Autodesk Inventor part; units mm, degrees
ref_plane "YZ Plane" through (0, 0, 0) normal (1, 0, 0) x (0, 1, 0)
ref_plane "XZ Plane" through (0, 0, 0) normal (0, 1, 0) x (-1, 0, 0)
ref_plane "XY Plane" through (0, 0, 0) normal (0, 0, 1) x (1, 0, 0)
sketch "Sketch1" plane through (0, 0, 0) normal (0, 1, 0) x (-1, 0, 0)
  line L0 (10.6592, 63.5) -> (-7.8828, 63.5)
  line L1 (-7.8828, 63.5) -> (-7.8828, -12.7)
  line L2 (-7.8828, -12.7) -> (10.6592, -12.7)
  line L3 (10.6592, 57.785) -> (-1.5328, 57.785)
  line L4 (-1.5328, 57.785) -> (-1.5328, 31.75)
  line L5 (-1.5328, 31.75) -> (10.6592, 31.75)
  line L6 (10.6592, 19.05) -> (-1.5328, 19.05)
  line L7 (-1.5328, 19.05) -> (-1.5328, -6.35)
  line L8 (-1.5328, -6.35) -> (10.6592, -6.35)
  line L9 (10.6592, -12.7) -> (10.6592, -6.35)
  line L10 (10.6592, 19.05) -> (10.6592, 31.75)
  line L11 (10.6592, 57.785) -> (10.6592, 63.5)
  point P0 (0, 0)
  dimension "d0" = 18.542
  dimension "d3" = 6.35
  dimension "d4" = 12.7
  dimension "d5" = 5.715
  dimension "d7" = 0
  dimension "d8" = 26.035
  dimension "d9" = 25.4
  dimension "d25" = 0
  dimension "d26" = 0
extrude "Extrusion1" add sketch "Sketch1" along normal blind 101.6
sketch "Sketch2" plane through (1.5328, 0, -6.35) normal (-1, 0, 0) x (0, 0, 1)
  line L0 (0, 0) -> (0, 101.6)
  line L1 (0, 0) -> (25.4, 0)
  point P0 (6.35, 0)
  point P1 (12.7, 25.4)
  point P2 (12.7, 50.8)
  point P3 (12.7, 76.2)
  dimension "d12" = 12.7
  dimension "d13" = 25.4
  dimension "d14" = 25.4
  dimension "d15" = 0
  dimension "d16" = 0
  dimension "d17" = 25.4
hole "Hole1" at (1.5328, 25.4, 6.35) at (1.5328, 50.8, 6.35) at (1.5328, 76.2, 6.35) direction (1, 0, 0) diameter 4.826 depth 25.4 tip angle 118
sketch "Sketch3" plane through (0, 101.6, 0) normal (0, 1, 0) x (1, 0, 0)
  line L0 (1.5328, -31.75) -> (-10.7917, -31.3196)
  line L1 (-10.7917, -31.3196) -> (-10.7917, -31.75)
  line L2 (-10.6592, -31.75) -> (1.5328, -31.75)
  line L3 (-10.7917, -31.75) -> (1.5328, -31.75)
  point P0 (0, 0)
  dimension "d27" = 2
extrude "Extrusion2" cut sketch "Sketch3" against normal blind 111.125
sketch "Sketch4" plane through (0, 101.6, 0) normal (0, 1, 0) x (1, 0, 0)
  line L0 (1.5328, -57.785) -> (-12.9577, -57.785)
  line L1 (-12.9577, -57.785) -> (-12.9577, -58.291)
  line L2 (-12.9577, -58.291) -> (1.5328, -57.785)
  point P0 (0, 0)
  dimension "d30" = 2
extrude "Extrusion3" cut sketch "Sketch4" against normal blind 119.0625
sketch "Sketch5" plane through (0, 101.6, 0) normal (0, 1, 0) x (1, 0, 0)
  line L0 (-10.6592, -63.5) -> (7.8828, -63.5)
  line L1 (7.8828, -63.5) -> (-13.0423, -62.7693)
  line L2 (-13.0423, -62.7693) -> (-13.0009, -63.5)
  line L3 (-13.0009, -63.5) -> (7.8828, -63.5)
  point P0 (0, 0)
  dimension "d33" = 2
extrude "Extrusion4" cut sketch "Sketch5" against normal blind 196.85
sketch "Sketch6" plane through (0, 101.6, 0) normal (0, 1, 0) x (1, 0, 0)
  line L0 (7.8828, 12.7) -> (-10.6592, 12.7)
  line L1 (7.8828, 12.7) -> (-16.8119, 12.7)
  line L2 (-16.8119, 12.7) -> (-16.8119, 11.8376)
  line L3 (7.8828, -63.5) -> (7.8828, 12.7)
  line L4 (-16.8119, 11.8376) -> (7.8828, 12.7)
  point P0 (0, 0)
  dimension "d36" = 2
extrude "Extrusion5" cut sketch "Sketch6" against normal blind 334.9625
sketch "Sketch8" plane through (1.5328, 0, -6.35) normal (-1, 0, 0) x (0, 0, 1)
  line L0 (0, 0) -> (25.4, 0)
  circle A0 centre (12.7, 25.4) radius 2.413
  circle A1 centre (12.7, 50.8) radius 2.413
  circle A2 centre (12.7, 76.2) radius 2.413
  line L1 (25.4, 0) -> (25.4, 101.6)
  line L2 (0, 0) -> (25.4, 0)
  line L3 (25.4, 0) -> (25.4, 101.6)
  line L4 (25.4, 101.6) -> (0, 101.6)
  line L5 (0, 101.6) -> (0, 0)
  circle A3 centre (12.7, 25.4) radius 2.413
  circle A4 centre (12.7, 50.8) radius 2.413
  circle A5 centre (12.7, 76.2) radius 2.413
  point P0 (6.35, 0)
extrude "Extrusion7" add sketch "Sketch8" along normal blind 1.1906
sketch "Sketch14" plane through (1.5328, 0, 31.75) normal (-1, 0, 0) x (0, 0, 1)
  circle A0 centre (14.2928, 23.4865) radius 3.5876
  circle A1 centre (14.2928, 70.9236) radius 3.7334
  point P0 (-31.75, 0)
extrude "Extrusion11" cut sketch "Sketch14" against normal blind 55.5625
sketch "Sketch15" plane through (-10.6592, 0, 19.05) normal (-1, 0, 0) x (0, 0, 1)
  line L0 (-46.1003, -15.0429) -> (50.4982, -15.0429)
  line L1 (50.4982, -15.0429) -> (50.4982, 3.175)
  line L2 (50.4982, 3.175) -> (-46.1003, 3.175)
  line L3 (-46.1003, 3.175) -> (-46.1003, -15.0429)
  line L4 (0, 0) -> (12.2742, 0)
  line L5 (-42.8623, 98.425) -> (49.6887, 98.425)
  line L6 (49.6887, 98.425) -> (49.6887, 110.1573)
  line L7 (49.6887, 110.1573) -> (-42.8623, 110.1573)
  line L8 (-42.8623, 110.1573) -> (-42.8623, 98.425)
  line L9 (0, 101.6) -> (12.2742, 101.6)
  point P0 (-19.05, 0)
  dimension "d55" = 3.175
  dimension "d56" = 3.175
extrude "Extrusion12" cut sketch "Sketch15" against normal blind 50.8
equation "\"d0\" = ElvDelWidth"
equation "\"d3\" = ElvDelFrontTabLength"
equation "\"d9\" = ElvBeamWidth"
equation "\"d10\" = ElvDelHeight"
equation "\"ElvBeamWidth\" = 25.4"
equation "\"ElvDelWidth\" = 18.542"
equation "\"ElvDelHeight\" = 101.6"
equation "\"ElvDelFrontTabLength\" = 6.35"
equation "\"ElvDelDepth\" = 6.35"
equation "\"d2\" = ElvDelDepth"
equation "\"ElvCrossBeamLength\" = 304.8"
equation "\"ElvFixedBeamLength\" = 990.6"
equation "\"ElvMiddleBeamLength\" = 990.6"
equation "\"ElvFrontBeamLength\" = 990.6"
equation "\"ElvEndEffectLength\" = 431.8"
equation "\"ElvWallWidth\" = 1.5875"
equation "\"ElvTopBeamLength\" = 457.2"
equation "\"ElvHoleFromFront\" = 25.4"
equation "\"ElvHoleFromMid\" = 38.1"
equation "\"ElvHoleFromFixed\" = 50.8"
equation "\"ElvHoleFromBottom\" = 38.1"
equation "\"ElvRivetPlateLength\" = 76.2"
equation "\"ElvDelMiddleTabLength\" = 6.35"
properties part number "ElvDelV6" material "Acetal Resin, White"
Design review of the part built by this model. Coordinates are the model's own, in mm. A direction names the side the tool comes from. Give positions to 0.01 mm unless a question says otherwise; leave off trailing zeros. Write each loop counter-clockwise with the first axis right and the second up, starting at its lowest first coordinate (ties: lowest second). Pieces come first, ordered by that corner, then holes. Notation, with made-up numbers: M 79.25,24.5 L 87.25,24.5 A26 ccw 87.25,58.5 Z; hole C 39,68.25 d10. An arc over 180 degrees is marked long. Return JSON: item names as keys, results as strings. Group by question number.
Item 1: Tool access review of faces 1 (the cylindrical face through (4.165, 27.541, 7.463)), 2 (the flat face through (-5, 50, -6.35)): name each direction out of +Z, -Z, +X, -X, +Y, -Y from which nothing blocks a thin tool from reaching the whole face with its end or side.
Item 2: The part is to be moulded in two halves that separate along Z. For faces 3 (the cylindrical face through (4.165, 78.556, 5.827)), 4 (the cylindrical face through (4.66, 67.28, 45.23)), 5 (the flat face through (1, 98.425, 25)), say which applies: pulls with the +Z half, pulls with the -Z half, needs draft (parallel to the pull), parting line crosses it, or undercut.
Item 3: Take a section at D-D (y = 15.5). Give the boundary of the cut face in (x, z) (3 decimals).
Item 4: Take a section at B-B (y = 76.2). Give the boundary of the cut face in (x, z) (3 decimals), plus the area to 3 significant figures.
Item 5: Clearance check with flat-ended pins moving along their axes: pin 1 Ø4 at (y, z) = (50.8, 6.35) entering from -X (3 decimals); pin 2 Ø5.5 at (x, y) = (-6.5, 31) entering from -Z; pin 3 Ø4 at (x, y) = (4, 40.5) entering from -Z; pin 4 Ø6 at (x, y) = (-9, 66) entering from +Z. State where each tip first meets the part, or that it passes through.
Item 6: Take a section at C-C (x = 5). Count the separate pieces of the cut face and the enclosed holes in it, plus the area to 3 significant figures.
Item 7: Take a section at A-A (z = 6.35). Give the boundary of the cut face in (x, y) (3 decimals).
Item 8: Wall thickness on line 1 along Y through (x, z) = (5, 6.35) (3 decimals); line 2 along Z through (x, y) = (-3, 24); line 3 along Z through (x, y) = (0, 74.5): over which ranges is each line inside the solid? List them lowest first.
Return value:
{
 "1": {"face 1": "+X, -X", "face 2": "-X, +Y, -Y"},
 "2": {"face 3": "undercut", "face 4": "undercut", "face 5": "needs draft"},
 "3": {"outline": "M -10.659,-12.052 L 7.883,-12.7 L 7.883,63.5 L -10.659,62.853 L -10.659,58.211 L 1.533,57.785 L 1.533,31.75 L -10.659,31.324 L -10.659,19.05 L 0.342,19.05 L 0.342,-6.35 L -10.659,-6.35 Z"},
 "4": {"outline": "M -10.659,-12.052 L 7.883,-12.7 L 7.883,3.937 L 0.342,3.937 L 0.342,-6.35 L -10.659,-6.35 Z; M -10.659,19.05 L 0.342,19.05 L 0.342,8.763 L 7.883,8.763 L 7.883,63.5 L -10.659,62.853 L -10.659,58.211 L 1.533,57.785 L 1.533,31.75 L -10.659,31.324 Z", "area": "762 mm2"},
 "5": {"pin 1": "passes through", "pin 2": "stops at z = -12.29", "pin 3": "stops at z = -12.63", "pin 4": "stops at z = 63.02"},
 "6": {"separate pieces": "1", "enclosed holes": "5", "area": "7,100 mm2"},
 "7": {"outline": "M 0.342,3.175 L 7.883,3.175 L 7.883,22.987 L 0.342,22.987 Z; M 0.342,27.813 L 7.883,27.813 L 7.883,48.387 L 0.342,48.387 Z; M 0.342,53.213 L 7.883,53.213 L 7.883,73.787 L 0.342,73.787 Z; M 0.342,78.613 L 7.883,78.613 L 7.883,98.425 L 0.342,98.425 Z"},
 "8": {"line 1": "y = 3.175 to 22.987, 27.813 to 48.387, 53.213 to 73.787, 78.613 to 98.425", "line 2": "z = -12.32 to -6.35, 19.05 to 31.59, 57.94 to 63.12", "line 3": "z = -12.42 to -6.35, 19.05 to 31.7, 57.84 to 63.22"}
}
